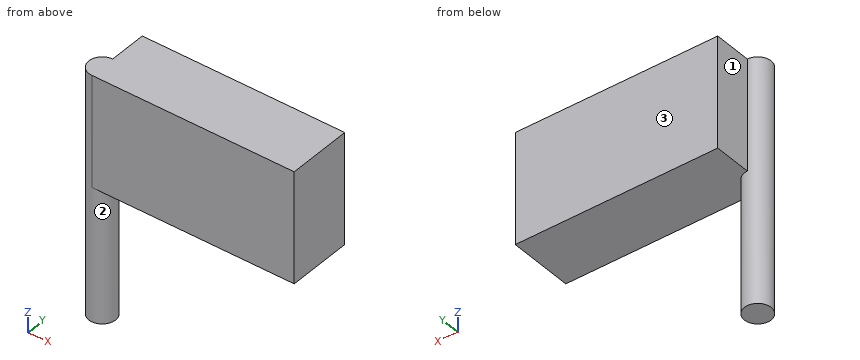
from build123d import *

# Parameters (mm, degrees)
CYLINDER_R     = 3
CYLINDER_DEPTH = 55
BOX_W          = 45.5
BOX_H          = 14.5
BOX_DEPTH      = 25


with BuildPart() as cylinder:
    # Cylinder → Cylinder (new body)
    with BuildSketch(Plane.XY):
        Circle(CYLINDER_R)
    extrude(amount=CYLINDER_DEPTH)


with BuildPart() as fusion:
    # Box → Box (new body)
    with BuildSketch(Plane(origin=(0, -3, 30), x_dir=(1, 0, 0), z_dir=(0, 0, 1))):
        with Locations((22.75, 7.25)):
            Rectangle(BOX_W, BOX_H)
    extrude(amount=BOX_DEPTH)

    # Fusion: union Cylinder
    add(cylinder.part)


solid = fusion.part
Geometry check sheet. Reference: the model listing, model coordinates, mm. Face numbers are marked on the shaded views. A direction names the side the tool comes from. Round coordinates to 2 decimals unless told otherwise and drop trailing zeros. Loops run counter-clockwise (first coordinate to the right, second up) from the corner with the lowest first, then second, coordinate; pieces in that order, holes last. Notation, with made-up numbers: (-27, 43.25) -> (31, 43.25) arc R18 cw to (31, 73.25) -> close; hole circle Ø7 at (-12, -12.75). An arc over 180 degrees is marked (long way). Answer as a JSON object with one key per item and string values. Group by question number.
Item 1: Cross-section at C-C, the plane x = 26. Record the cut outline in (y, z), plus the area to 4 significant figures.
Item 2: Cross-section at A-A, the plane y = 0. Record the cut outline in (x, z).
Item 3: Set-up check for the marked faces 1, 2 and 3: record each of +Z, -Z, +X, -X, +Y, -Y from which the full face is reachable in a straight line by a thin tool's end or side.
Item 4: Thickness scan on line 1 along Z through (x, y) = (32, 3.25); line 2 along X through (y, z) = (6.5, 45.5); line 3 along X through (y, z) = (0.25, 6). Record the ranges inside material, lowest first.
Item 5: Cross-section at B-B, the plane z = 36. Record the cut outline in (x, y).
Item 6: Cross-section at D-D, the plane y = 4.5. Record the cut outline in (x, z), plus the area to 3 significant figures.
Item 7: Depth check by flat-ended pin: pin 1 Ø1 at (x, z) = (12, 29) entering from -Y; pin 2 Ø2.5 at (y, z) = (8.5, 39) entering from -X; pin 3 Ø4.5 at (x, y) = (19, 6.5) entering from -Z. Enter the tip coordinate at first touch or a pass-through.
Determined:
{
 "1": {"outline": "(-3, 30) -> (11.5, 30) -> (11.5, 55) -> (-3, 55) -> close", "area": "362.5 mm²"},
 "2": {"outline": "(-3, 0) -> (3, 0) -> (3, 30) -> (45.5, 30) -> (45.5, 55) -> (-3, 55) -> close"},
 "3": {"face 1": "+Z, -Z, -X, +Y", "face 2": "-Z", "face 3": "+Z, -Z, +X, -X, +Y"},
 "4": {"line 1": "z = 30 to 55", "line 2": "x = 0 to 45.5", "line 3": "x = -2.99 to 2.99"},
 "5": {"outline": "(0, -3) -> (45.5, -3) -> (45.5, 11.5) -> (0, 11.5) -> (0, 3) arc R3 ccw to start"},
 "6": {"outline": "(0, 30) -> (45.5, 30) -> (45.5, 55) -> (0, 55) -> close", "area": "1,140 mm²"},
 "7": {"pin 1": "passes through", "pin 2": "stops at x = 0", "pin 3": "stops at z = 30"}
}
